from build123d import *

# Parameters (mm, degrees)
F0_R     = 1.5875
F1_DEPTH = 3.048


with BuildPart() as f1:
    # F0 (on Front) → F1 (new body)
    with BuildSketch(Plane.XZ):
        with BuildLine():
            ThreePointArc((-50.5042680437, 63.6216618954), (-47.1542651109, 57.382604112), (-40.4239670527, 55.1800034394))
            ThreePointArc((-40.4239670527, 55.1800034394), (-34.0896459808, 58.1709562478), (-31.5138232961, 64.6851376731))
            ThreePointArc((-31.5138232961, 64.6851376731), (-31.5163410034, 64.9041262217), (-31.5238927941, 65.1229990015))
            ThreePointArc((-31.5238927941, 65.1229990015), (-41.7898995149, 74.1804791368), (-50.5042680437, 63.6216618954))
        make_face()
        with BuildLine():
            ThreePointArc((-37.8638232961, 64.6851376731), (-38.7224308577, 62.5137438647), (-40.833871215, 61.5167595952))
            ThreePointArc((-40.833871215, 61.5167595952), (-43.3552157345, 66.8565314815), (-37.8638232961, 64.6851376731))
        make_face(mode=Mode.SUBTRACT)
        with BuildLine():
            ThreePointArc((-31.5138232961, 64.6851376731), (-34.0896459808, 58.1709562478), (-40.4239670527, 55.1800034394))
            Line((-40.4239670527, 55.1800034394), (-38.7843504035, 29.8329788163))
            ThreePointArc((-38.7843504035, 29.8329788163), (-28.0623580194, 26.5600707626), (-22.1761003167, 17.0193675354))
            Line((-22.1761003167, 17.0193675354), (-31.5238927941, 65.1229990015))
            ThreePointArc((-31.5238927941, 65.1229990015), (-31.5163410034, 64.9041262217), (-31.5138232961, 64.6851376731))
        make_face()
        with BuildLine():
            Line((-38.7843504035, 29.8329788163), (-40.4239670527, 55.1800034394))
            ThreePointArc((-40.4239670527, 55.1800034394), (-47.1542651109, 57.382604112), (-50.5042680437, 63.6216618954))
            Line((-50.5042680437, 63.6216618954), (-53.60245848, 15.0006146799))
            ThreePointArc((-53.60245848, 15.0006146799), (-48.9903060277, 25.2110101047), (-38.7843504035, 29.8329788163))
        make_face()
        with Locations((-43.7214151025, 50.5162884269)):
            Circle(F0_R, mode=Mode.SUBTRACT)
        with BuildLine():
            ThreePointArc((-22.1761003167, 17.0193675354), (-28.0623580194, 26.5600707626), (-38.7843504035, 29.8329788163))
            Line((-38.7843504035, 29.8329788163), (-37.9645420789, 17.1594665048))
            ThreePointArc((-37.9645420789, 17.1594665048), (-35.5881961894, 16.3074808653), (-34.5845899978, 13.9910884269))
            ThreePointArc((-34.5845899978, 13.9910884269), (-35.4431975594, 11.8196946185), (-37.5546379166, 10.822710349))
            Line((-37.5546379166, 10.822710349), (-36.7348295921, -1.8508019626))
            ThreePointArc((-36.7348295921, -1.8508019626), (-26.1776278056, 3.1341193848), (-21.8845899978, 13.9910884269))
            ThreePointArc((-21.8845899978, 13.9910884269), (-21.9576356299, 15.5122271964), (-22.1761003167, 17.0193675354))
        make_face()
        with BuildLine():
            Line((-37.9645420789, 17.1594665048), (-38.7843504035, 29.8329788163))
            ThreePointArc((-38.7843504035, 29.8329788163), (-48.9903060277, 25.2110101047), (-53.60245848, 15.0006146799))
            ThreePointArc((-53.60245848, 15.0006146799), (-53.6146740156, 13.1961445378), (-53.4220280351, 11.4019457641))
            ThreePointArc((-53.4220280351, 11.4019457641), (-47.6324939367, 1.5596205806), (-36.7348295921, -1.8508019626))
            Line((-36.7348295921, -1.8508019626), (-37.5546379166, 10.822710349))
            ThreePointArc((-37.5546379166, 10.822710349), (-40.9279680757, 13.7861363457), (-37.9645420789, 17.1594665048))
        make_face()
        with BuildLine():
            Line((-21.7838038896, 15.0006146799), (-22.1761003167, 17.0193675354))
            ThreePointArc((-22.1761003167, 17.0193675354), (-21.9576356299, 15.5122271964), (-21.8845899978, 13.9910884269))
            ThreePointArc((-21.8845899978, 13.9910884269), (-26.1776278056, 3.1341193848), (-36.7348295921, -1.8508019626))
            Line((-36.7348295921, -1.8508019626), (-34.3163950346, -39.2376632816))
            ThreePointArc((-34.3163950346, -39.2376632816), (-26.9550807978, -41.7434983128), (-23.5217385257, -48.7206264712))
            Line((-23.5217385257, -48.7206264712), (2.7757995208, -47.0195241977))
            ThreePointArc((2.7757995208, -47.0195241977), (5.0392904077, -40.9396385387), (11.0821216178, -38.5790048126))
            Line((11.0821216178, -38.5790048126), (-15.3970316035, -37.2918863845))
            ThreePointArc((-15.3970316035, -37.2918863845), (-20.8399623866, -34.7574770434), (-22.9584246143, -29.1395731632))
            Line((-22.9584246143, -29.1395731632), (-21.7838038896, 15.0006146799))
        make_face()
        with BuildLine():
            ThreePointArc((-36.7348295921, -1.8508019626), (-47.6324939367, 1.5596205806), (-53.4220280351, 11.4019457641))
            Line((-53.4220280351, 11.4019457641), (-43.6992026963, -50.9420463215))
            ThreePointArc((-43.6992026963, -50.9420463215), (-41.5877946429, -43.0216036117), (-34.3163950346, -39.2376632816))
            Line((-34.3163950346, -39.2376632816), (-36.7348295921, -1.8508019626))
        make_face()
        with BuildLine():
            ThreePointArc((-34.3163950346, -39.2376632816), (-41.5877946429, -43.0216036117), (-43.6992026963, -50.9420463215))
            ThreePointArc((-43.6992026963, -50.9420463215), (-40.4647037817, -56.9216085968), (-34.1837836398, -59.5229909995))
            Line((-34.1837836398, -59.5229909995), (-30.9047285274, -59.1555864326))
            ThreePointArc((-30.9047285274, -59.1555864326), (-25.5604023993, -55.5094361321), (-23.5005483749, -49.3764731309))
            ThreePointArc((-23.5005483749, -49.3764731309), (-23.5058472944, -49.0483786843), (-23.5217385257, -48.7206264712))
            Line((-23.5217385257, -48.7206264712), (-30.492170297, -49.1715210497))
            ThreePointArc((-30.492170297, -49.1715210497), (-30.4872042872, -49.2739436163), (-30.4855483749, -49.3764731309))
            ThreePointArc((-30.4855483749, -49.3764731309), (-35.8319421833, -51.6928655693), (-33.865500456, -46.208095053))
            Line((-33.865500456, -46.208095053), (-34.3163950346, -39.2376632816))
        make_face()
        with BuildLine():
            Line((-30.9047285274, -59.1555864326), (-34.1837836398, -59.5229909995))
            ThreePointArc((-34.1837836398, -59.5229909995), (-32.5292416046, -59.4732916888), (-30.9047285274, -59.1555864326))
        make_face()
        with BuildLine():
            Line((2.7757995208, -47.0195241977), (-23.5217385257, -48.7206264712))
            ThreePointArc((-23.5217385257, -48.7206264712), (-23.5058472944, -49.0483786843), (-23.5005483749, -49.3764731309))
            ThreePointArc((-23.5005483749, -49.3764731309), (-25.5604023993, -55.5094361321), (-30.9047285274, -59.1555864326))
            Line((-30.9047285274, -59.1555864326), (11.5805781298, -54.3952834932))
            ThreePointArc((11.5805781298, -54.3952834932), (5.5996188736, -52.5918144379), (2.7757995208, -47.0195241977))
        make_face()
        with BuildLine():
            ThreePointArc((18.6342447155, -46.5071439948), (16.4440412718, -41.0324304367), (11.0821216178, -38.5790048126))
            ThreePointArc((11.0821216178, -38.5790048126), (5.0392904077, -40.9396385387), (2.7757995208, -47.0195241977))
            ThreePointArc((2.7757995208, -47.0195241977), (5.5996188736, -52.5918144379), (11.5805781298, -54.3952834932))
            ThreePointArc((11.5805781298, -54.3952834932), (16.6136414518, -51.7981022504), (18.6342447155, -46.5071439948))
        make_face()
        with BuildLine():
            ThreePointArc((13.8717447155, -46.5071439948), (10.7992742301, -49.6804880825), (7.5283666376, -46.712096076))
            ThreePointArc((7.5283666376, -46.712096076), (10.594215201, -43.3337999072), (13.8717447155, -46.5071439948))
        make_face(mode=Mode.SUBTRACT)
    extrude(amount=F1_DEPTH)


solid = f1.part
Source: CAD feature listing. Evaluate the final solid. Frame: model axes, mm. A direction names the side the tool comes from. Coordinates: 2 decimals unless noted, no trailing zeros. Loops run counter-clockwise (first coordinate to the right, second up) from the corner with the lowest first, then second, coordinate; pieces in that order, holes last. Notation, with made-up numbers: (37.5, 74.25) - (96.5, 74.25) arc R19 ccw to (96.5, 100.25) - close; hole circle Ø10 at (-3, -12). An arc over 180 degrees is marked (long way). One line per item, written item: value. Start each with the question number.
1. Section B-B (z = 28). Return the cut outline in (x, y), and give its area (3 significant figures).
2. Set-up query: faces 1 (the cylindrical face through (-53.616, -1.503, 13.221)), 2 (the flat face through (-26.958, -1.503, -48.943)), 3 (the cylindrical face through (-20.8, -1.5, -34.8)). Return all of +Z, -Z, +X, -X, +Y, -Y with unobstructed straight access to the full face (end or side cutting, diameter ignored); none if empty.
3. Section A-A (y = -1.45). State how many separate pieces and enclosed holes the cut face has, and give its area (3 significant figures).
4. Section C-C (x = -9). Return the cut outline in (y, z), and give its area (3 significant figures).
5. Ray query, L1, parallel to Z at x = -41, y = -2.45; L2, parallel to X at y = -1.55, z = -42.5; L3, parallel to X at y = -2.15, z = -50. Return the intervals inside material, ascending.
Verdict:
1. outline: (-52.77, -3.05) - (-24.31, -3.05) - (-24.31, 0) - (-52.77, 0) - close
1. area: 86.8 mm2
2. face 1: -X, +Y, -Y
2. face 2: +Y, -Y
2. face 3: +X, +Y, -Y
3. separate pieces: 1
3. enclosed holes: 5
3. area: 3,820 mm2
4. outline: (-3.05, -56.7) - (0, -56.7) - (0, -37.6) - (-3.05, -37.6) - close
4. area: 58.2 mm2
5. L1: z = -56.4 to 61.51, 67.86 to 74.21
5. L2: x = -45.02 to -34.11, -26.18 to 17.55
5. L3: x = -43.85 to -36.77, -30.55 to 17.82
